Autodesk Inventor part; units mm, degrees
ref_plane "YZ Plane" through (0, 0, 0) normal (1, 0, 0) x (0, 1, 0)
ref_plane "XZ Plane" through (0, 0, 0) normal (0, 1, 0) x (-1, 0, 0)
ref_plane "XY Plane" through (0, 0, 0) normal (0, 0, 1) x (1, 0, 0)
sketch "Skizze1" plane through (0, 0, 0) normal (0, 0, 1) x (1, 0, 0)
  line L0 (-35.5, 36) -> (35.5, 36)
  line L1 (35.5, 36) -> (35.5, -20)
  line L2 (35.5, -20) -> (-35.5, -20)
  line L3 (-35.5, -20) -> (-35.5, 36)
  circle A0 centre (0, 0) radius 4.25
  circle A1 centre (-27, 0) radius 6.125
  circle A2 centre (27, 0) radius 6.125
  point P0 (0, -20)
  point P1 (35.5, 8)
  dimension "d0" = 71
  dimension "d1" = 56
  dimension "d2" = 20
  dimension "d3" = 35.5
  dimension "d4" = 8.5
  dimension "d5" = 12.25
  dimension "d6" = 12.25
  dimension "d7" = 27
  dimension "d8" = 27
extrude "Extrusion1" add sketch "Skizze1" along normal blind 9
sketch "Skizze2" plane through (0, 0, 9) normal (0, 0, 1) x (1, 0, 0)
  arc A0 (-22.5, 30) -> (-11.5, 30) centre (-17, 30) ccw
  arc A1 (0, 30) -> (22, 30) centre (11, 30) ccw
  line L0 (35.5, 36) -> (-35.5, 36)
  line L1 (-35.5, 36) -> (-35.5, -20)
  line L2 (35.5, -20) -> (35.5, 36)
  line L3 (-22.5, 30) -> (-22.5, 36)
  line L4 (-11.5, 30) -> (-11.5, 36)
  line L5 (0, 30) -> (0, 36)
  line L6 (22, 30) -> (22, 36)
  point P0 (0, 0)
  dimension "d11" = 11
  dimension "d12" = 22
  dimension "d13" = 6
  dimension "d14" = 6
  dimension "d15" = 18.5
  dimension "d16" = 24.5
extrude "Extrusion2" cut sketch "Skizze2" against normal blind 1.67
sketch "Skizze3" plane through (0, 0, 9) normal (0, 0, 1) x (1, 0, 0)
  line L0 (-22.5, 36) -> (-35.5, 36)
  line L1 (35.5, 36) -> (35.5, -20)
  line L2 (35.5, -20) -> (-35.5, -20)
  line L3 (-35.5, -20) -> (-35.5, 36)
  circle A0 centre (-27, 0) radius 6.125
  circle A1 centre (0, 0) radius 4.25
  circle A2 centre (27, 0) radius 6.125
  circle A3 centre (27, 0) radius 6.125
  circle A4 centre (-27, 0) radius 6.125
  arc A5 (-19.5, 30) -> (-14.5, 30) centre (-17, 30) ccw
  arc A6 (-22.5, 30) -> (-11.5, 30) centre (-17, 30) ccw
  arc A7 (4.5, 30) -> (17.5, 30) centre (11, 30) ccw
  arc A8 (0, 30) -> (22, 30) centre (11, 30) ccw
  line L4 (-19.5, 30) -> (-19.5, 36)
  line L5 (-14.5, 30) -> (-14.5, 36)
  line L6 (4.5, 30) -> (4.5, 36)
  line L7 (17.5, 30) -> (17.5, 36)
  line L8 (17.5, 36) -> (35.5, 36)
  line L9 (-35.5, 36) -> (-19.5, 36)
  line L10 (-14.5, 36) -> (4.5, 36)
  dimension "d19" = 71
  dimension "d20" = 56
  dimension "d21" = 12.25
  dimension "d22" = 12.25
  dimension "d23" = 0
  dimension "d24" = 0
  dimension "d25" = 5
  dimension "d26" = 0
  dimension "d27" = 13
  dimension "d28" = 0
  dimension "d29" = 0
  dimension "d30" = 0
extrude "Extrusion3" add sketch "Skizze3" along normal blind 11
fillet "Rundung1" radius 6 2 edges at (35.5, 36, 10) (-35.5, 36, 10)
fillet "Rundung2" radius 3 2 edges at (-35.5, -20, 10) (35.5, -20, 10)
sketch "Skizze4" plane through (0, 0, 20) normal (0, 0, 1) x (1, 0, 0)
  line L0 (-32.5, -20) -> (32.5, -20)
  line L1 (-35.5, 30) -> (-35.5, -17)
  line L2 (-27.5, -20) -> (-35.5, -20)
  line L3 (-35.5, -20) -> (-35.5, -7)
  line L4 (-35.5, -7) -> (-27.5, -7)
  line L5 (-27.5, -7) -> (-27.5, -20)
  line L6 (27.5, -20) -> (35.5, -20)
  line L7 (35.5, -20) -> (35.5, -7)
  line L8 (35.5, -7) -> (27.5, -7)
  line L9 (27.5, -7) -> (27.5, -20)
  line L10 (35.5, -17) -> (35.5, 30)
  point P0 (0, 0)
  point P1 (-35.5, -17)
  dimension "d35" = 8
  dimension "d36" = 13
  dimension "d37" = 8
  dimension "d38" = 0
sketch "Skizze5" plane through (0, 0, 0) normal (0, 0, -1) x (-1, 0, 0)
  line L0 (32.5, -20) -> (-32.5, -20)
  line L1 (35.5, 30) -> (35.5, -17)
  line L2 (27.5, -20) -> (35.5, -20)
  line L3 (35.5, -20) -> (35.5, -7)
  line L4 (35.5, -7) -> (27.5, -7)
  line L5 (27.5, -7) -> (27.5, -20)
  line L6 (-35.5, -14) -> (-35.5, -7)
  line L7 (-35.5, -7) -> (-27.5, -7)
  line L8 (-27.5, -7) -> (-27.5, -20)
  line L9 (-27.5, -20) -> (-35.5, -20)
  line L10 (-35.5, -20) -> (-35.5, -7)
  point P0 (0, 0)
  point P1 (29.5, -20)
  point P2 (-29.5, -20)
  point P3 (35.5, -14)
  point P4 (29.5, -20)
  point P5 (35.5, -14)
  point P6 (-29.5, -20)
  dimension "d42" = 13
  dimension "d43" = 8
  dimension "d44" = 8
extrude "Extrusion5" add sketch "Skizze5" along normal blind 10
fillet "Rundung4" radius 6 2 edges at (-35.5, -20, -5) (35.5, -20, -5)
sketch "Skizze6" plane through (0, 0, 0) normal (0, 0, -1) x (-1, 0, 0)
  line L0 (6.5705, -3.7459) -> (0.0412, -7.5632)
  line L1 (0.0412, -7.5632) -> (-6.5293, -3.8173)
  line L2 (-6.5293, -3.8173) -> (-6.5705, 3.7459)
  line L3 (-6.5705, 3.7459) -> (-0.0412, 7.5632)
  line L4 (-0.0412, 7.5632) -> (6.5293, 3.8173)
  line L5 (6.5293, 3.8173) -> (6.5705, -3.7459)
  point P0 (0, 0)
  point P1 (0, 0)
  point P2 (-6.5499, -0.0357)
  dimension "d48" = 13.1
extrude "Extrusion6" cut sketch "Skizze6" against normal blind 13.5
sketch "Skizze7" plane through (0, 0, 7.33) normal (0, 0, 1) x (1, 0, 0)
  arc A0 (-22.5, 30) -> (-11.5, 30) centre (-17, 30) ccw
  line L0 (-22.5, 30) -> (-22.5, 36)
  line L1 (-11.5, 36) -> (-11.5, 30)
  line L2 (-22.5, 36) -> (-11.5, 36)
  point P0 (0, 0)
extrude "Extrusion7" add sketch "Skizze7" along normal blind 0.4
sketch "Skizze8" plane through (0, 0, 7.73) normal (0, 0, 1) x (1, 0, 0)
  arc A0 (-22.5, 30) -> (-11.5, 30) centre (-17, 30) ccw
  arc A1 (-21.6, 30) -> (-12.4, 30) centre (-17, 30) ccw
  line L0 (-21.6, 30) -> (-21.6, 36)
  line L1 (-11.5, 36) -> (-22.5, 36)
  line L2 (-12.4, 30) -> (-12.4, 36)
  line L3 (-22.5, 30) -> (-22.5, 36)
  line L4 (-11.5, 36) -> (-11.5, 30)
  line L5 (4.5, 36) -> (-14.5, 36)
  line L6 (-19.5, 36) -> (-29.5, 36)
  point P0 (0, 0)
  dimension "d53" = 9.2
extrude "Extrusion8" add sketch "Skizze8" along normal blind 1.27 contours L3 L1 L0 A1 L2 L4 A0
sketch "Skizze9" plane through (0, 0, 20) normal (0, 0, 1) x (1, 0, 0)
  arc A0 (0, 30) -> (22, 30) centre (11, 30) ccw
  line L0 (2.75, 30) -> (2.75, 36)
  line L1 (0, 36) -> (22, 36)
  line L2 (19.25, 30) -> (19.25, 36)
  arc A1 (2.75, 30) -> (19.25, 30) centre (11, 30) ccw
  point P0 (0, 0)
extrude "Extrusion9" cut sketch "Skizze9" against normal blind 4
sketch "Skizze10" plane through (0, 0, 16) normal (0, 0, 1) x (1, 0, 0)
  arc A0 (0, 30) -> (22, 30) centre (11, 30) ccw
  line L0 (-1.8, 30) -> (-1.8, 36)
  line L1 (0, 36) -> (22, 36)
  line L2 (2.75, 36) -> (-14.5, 36)
  line L3 (29.5, 36) -> (19.25, 36)
  line L4 (23.8, 30) -> (23.8, 36)
  arc A1 (-1.8, 30) -> (23.8, 30) centre (11, 30) ccw
  point P0 (0, 0)
extrude "Extrusion10" cut sketch "Skizze10" against normal blind 1.67
properties part number "Guideteil_Spritzenpumpe001"
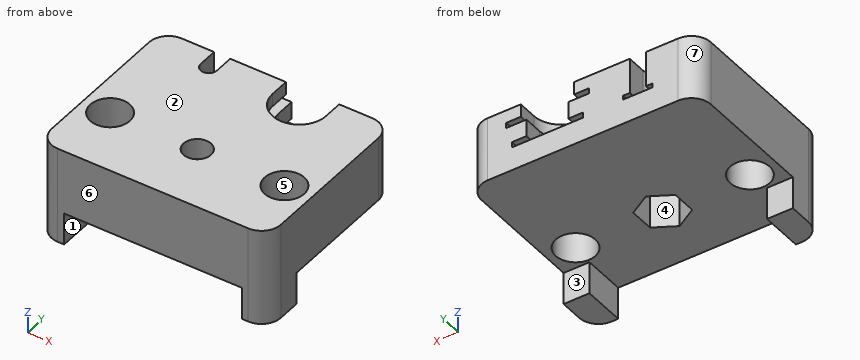
Work out the finished part from the listing and answer in its coordinate system (mm). Face numbers are marked on the shaded views. A direction names the side the tool comes from. Coordinates: 2 decimals unless noted, no trailing zeros. Loops run counter-clockwise (first coordinate to the right, second up) from the corner with the lowest first, then second, coordinate; pieces in that order, holes last. Notation, with made-up numbers: (11.25, 34.25) -> (25.25, 34.25) arc R17 ccw to (25.25, 56.25) -> close; hole circle Ø9 at (-14.75, 4). An arc over 180 degrees is marked (long way). Write each question's results on one line, items separated by ' | '. Start each with the question number.
1) For the marked faces 1, 2 and 3, determine the directions among +Z, -Z, +X, -X, +Y, -Y from which every point of the face is accessible in a straight line to the end or side of a thin tool.
2) The mould has two halves that part along X. Classify the marked faces 4, 5, 6 and 7: pulls with the +X half, pulls with the -X half, needs draft (parallel to the pull), parting line crosses it, or undercut.
3) Find section C-C on x = -17. Determine the outline of the cut face in (y, z).
4) Flat-ended cylindrical pins translate along their axes: P1, Ø8, axis at x = -3, z = -7, coming from the -Y side; P2, Ø17, axis at x = -17, y = -4, coming from the -Z side; P3, Ø1.6, axis at y = 34, z = 13, coming from the -X side; P4, Ø1.8, axis at y = 34.5, z = 8.5, coming from the +X side. Find the tip coordinate at first contact, or state that the pin passes through.
5) Find section A-A on z = -7.5. Determine the outline of the cut face in (x, y).
6) Consider line 1 along Y through (x, z) = (0, 18); line 2 along Y through (x, z) = (-27, 7.25) (3 decimals); line 3 along Z through (x, y) = (-6, 23). Determine where each line is inside the solid, lowest interval first.
7) Find section D-D on y = 2. Determine the outline of the cut face in (x, z), then the cut area to 3 significant figures.
8) Find section B-B on z = 11. Count the separate pieces of the cut face and the enclosed holes in it, then the cut area to 3 significant figures.
Response values:
1) face 1: -Z, +Y, -Y | face 2: +Z, +X, -X, +Y, -Y | face 3: -Z, +X, -X, +Y
2) face 4: undercut | face 5: undercut | face 6: needs draft | face 7: pulls with the -X half
3) outline: (-20, 0) -> (36, 0) -> (36, 7.73) -> (25.4, 7.73) -> (25.4, 9) -> (27.5, 9) -> (27.5, 20) -> (-20, 20) -> close
4) P1: passes through | P2: stops at z = 0 | P3: stops at x = -34.58 | P4: stops at x = 34.3
5) outline: (-35.5, -14) arc R6 ccw to (-29.5, -20) -> (-27.5, -20) -> (-27.5, -7) -> (-35.5, -7) -> close; (27.5, -20) -> (29.5, -20) arc R6 ccw to (35.5, -14) -> (35.5, -7) -> (27.5, -7) -> close
6) line 1: y = -20 to -4.25, 4.25 to 36 | line 2: y = -20 to -6.125, 6.125 to 36 | line 3: z = 0 to 20
7) outline: (-35.5, 0) -> (-32.79, 0) -> (-32.79, 20) -> (-35.5, 20) -> close; (-21.21, 0) -> (-6.54, 0) -> (-6.54, 13.5) -> (-3.75, 13.5) -> (-3.75, 20) -> (-21.21, 20) -> close; (3.75, 13.5) -> (6.56, 13.5) -> (6.56, 0) -> (21.21, 0) -> (21.21, 20) -> (3.75, 20) -> close; (32.79, 0) -> (35.5, 0) -> (35.5, 20) -> (32.79, 20) -> close | area: 731 mm^2
8) separate pieces: 1 | enclosed holes: 3 | area: 3,380 mm^2
